Design review of the part built by this model. Coordinates are the model's own, in mm. Give positions to 0.01 mm unless a question says otherwise; leave off trailing zeros. Write each loop counter-clockwise with the first axis right and the second up, starting at its lowest first coordinate (ties: lowest second). Pieces come first, ordered by that corner, then holes. Notation, with made-up numbers: (62.25, -33) - (111.25, -33) arc R29 cw to (111.25, -6) - close; hole circle Ø4 at (83.25, 41.5). An arc over 180 degrees is marked (long way). Use a Markdown table: item, result. Add a question column.
```python
from build123d import *

# Parameters (mm, degrees)
SKETCH1_R           = 1.65
BOSS_EXTRUDE1_DEPTH = 3.2
SKETCH2_W           = 4
SKETCH2_H           = 12
BOSS_EXTRUDE2_DEPTH = 3.2
FILLET1_R           = 1.5


with BuildPart() as part:
    # Sketch1 → Boss-Extrude1 (new body)
    with BuildSketch(Plane.XY):
        with BuildLine():
            Line((1.830127019, -31.504464167), (35.605117766, -51.004464167))
            Line((35.605117766, -51.004464167), (48.732545217, -54.648197122))
            ThreePointArc((48.732545217, -54.648197122), (49.6052046, -54.480696676), (50, -53.68462671))
            Line((50, -53.68462671), (50, 44))
            Line((50, 44), (48.060403212, 55))
            Line((48.060403212, 55), (46, 55))
            Line((46, 55), (0, -24.674337148))
            ThreePointArc((0, -24.674337148), (-0.499502113, -28.468432374), (1.830127019, -31.504464167))
        make_face()
        with Locations((38, -5)):
            Circle(SKETCH1_R, mode=Mode.SUBTRACT)
        Polygon((18.88414205, -7.96604366), (32.88414205, 16.282667646), (35.534179786, 14.752667646), (21.534179786, -9.49604366), align=None, mode=Mode.SUBTRACT)
    extrude(amount=BOSS_EXTRUDE1_DEPTH)

    # Sketch2 → Boss-Extrude2 (add)
    with BuildSketch(Plane.XY.offset(3.2)):
        with Locations((52, 26)):
            Rectangle(SKETCH2_W, SKETCH2_H)
    extrude(amount=-BOSS_EXTRUDE2_DEPTH)

    # Fillet1
    fillet1_edges = [part.edges().sort_by_distance(p)[0] for p in [
        (54, 32, 1.6),
        (54, 20, 1.6),
    ]]
    fillet(fillet1_edges, radius=FILLET1_R)


solid = part.part
```
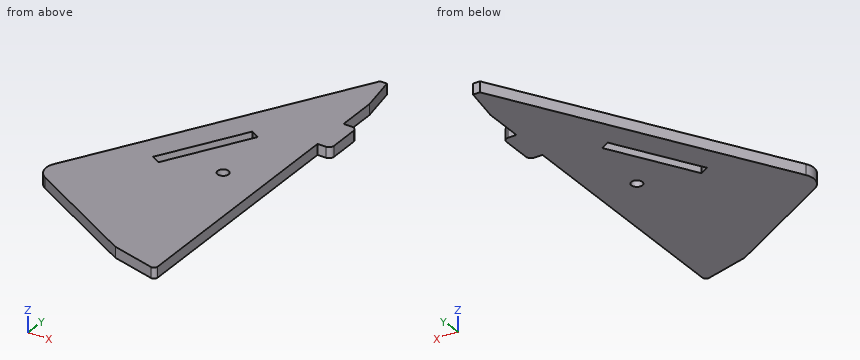
(1) Add section B-B (x = 38). State the section outline as (y, z) points.
(2) Insertion check: pin 1 (1 mm diameter, centred on x = 41.5, z = 1.5, fed in from +Y); pin 2 (5.5 mm diameter, centred on x = 38, y = -5, fed in from +Z); pin 3 (1.6 mm diameter, centred on y = 38, z = 1.5, fed in from +X); pin 4 (1 mm diameter, centred on x = 18, z = 1, fed in from -Y). Each pin has a flat end and moves straight along its axis. Give the tip position at first contact, or say it passes through.
(3) Add section D-D (x = 6.5). State the section outline as (y, z) points, and give its area (3 significant figures).
(4) Add section C-C (y = 1). State the section outline as (x, z) points, and give its area (3 significant figures).
(5) Add section A-A (z = 1.1). State the section outline as (x, y) points, and give its area (3 significant figures).
(6) For line 1 along Y through (x, z) = (38, 2.45); line 2 along Y through (x, z) = (26.5, 2.15) (3 decimals); line 3 along X through (y, z) = (2, 0.75), list the stretches that pass through material, from the lowest coordinate up.
Answers follow:
| question | item | result |
|---|---|---|
| 1 | outline | (-51.67, 0) - (-6.65, 0) - (-6.65, 3.2) - (-51.67, 3.2) - close; (-3.35, 0) - (41.14, 0) - (41.14, 3.2) - (-3.35, 3.2) - close |
| 2 | pin 1 | y = 48.07 |
| 2 | pin 2 | z = 3.2 |
| 2 | pin 3 | x = 50 |
| 2 | pin 4 | y = -41.13 |
| 3 | outline | (-34.2, 0) - (-13.42, 0) - (-13.42, 3.2) - (-34.2, 3.2) - close |
| 3 | area | 66.5 mm^2 |
| 4 | outline | (14.82, 0) - (24.06, 0) - (24.06, 3.2) - (14.82, 3.2) - close; (27.59, 0) - (50, 0) - (50, 3.2) - (27.59, 3.2) - close |
| 4 | area | 101 mm^2 |
| 5 | outline | (0, -24.67) arc R5 ccw to (1.83, -31.5) - (35.61, -51) - (48.73, -54.65) arc R1 ccw to (50, -53.68) - (50, 20) - (52.5, 20) arc R1.5 ccw to (54, 21.5) - (54, 30.5) arc R1.5 ccw to (52.5, 32) - (50, 32) - (50, 44) - (48.06, 55) - (46, 55) - close; hole (18.88, -7.97) - (21.53, -9.5) - (35.53, 14.75) - (32.88, 16.28) - close; hole circle Ø3.3 at (38, -5) |
| 5 | area | 3,070 mm^2 |
| 6 | line 1 | -51.67 to -6.65, -3.35 to 41.14 |
| 6 | line 2 | -45.748 to -0.895, 5.225 to 21.225 |
| 6 | line 3 | 15.4 to 24.64, 28.17 to 50 |
